```python
from build123d import *

# Parameters (mm, degrees)
SKETCH_1_W      = 60
SKETCH_1_H      = 48
EXTRUDE_1_DEPTH = 36
EXTRUDE_2_REACH = 96.488
SKETCH_2_R      = 10


with BuildPart() as part:
    # 草图1 → 凸台-拉伸1 (new body)
    with BuildSketch(Plane(origin=(0, 0, 0), x_dir=(1, 0, 0), z_dir=(0, 1, 0))):
        Rectangle(SKETCH_1_W, SKETCH_1_H)
    extrude(amount=EXTRUDE_1_DEPTH)

    # 草图2 → 凸台-拉伸2 (add, up to next)
    with BuildSketch(Plane(origin=(54, 0, 0), x_dir=(0, 0, -1), z_dir=(1, 0, 0)), mode=Mode.PRIVATE) as extrude_2_sk1:
        with Locations((0, 18)):
            Circle(SKETCH_2_R)
    extrude_2_tool1 = extrude(extrude_2_sk1.sketch, amount=-EXTRUDE_2_REACH, mode=Mode.PRIVATE) - part.part
    add(extrude_2_tool1.solids().sort_by_distance((54, 18, 0))[0])


solid = part.part
```
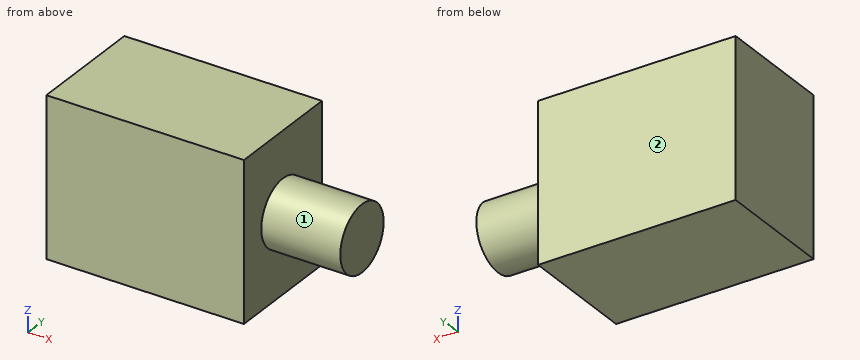
Geometry check sheet. Reference: the model listing, model coordinates, mm. Face numbers are marked on the shaded views. A direction names the side the tool comes from. Round coordinates to 2 decimals unless told otherwise and drop trailing zeros. Order: outer loops, then holes, each group sorted by start corner. A loop starts at its lowest first (then second) coordinate and runs counter-clockwise, first axis right, second up. Notation, with made-up numbers: (-12.5, -28) - (36.5, -28) arc R27 cw to (36.5, -4) - close; hole circle Ø7 at (36.5, 77). An arc over 180 degrees is marked (long way). Use a Markdown table: item, result. Add a question column.
1) Section check A-A (z = 0). Record the cut outline in (x, y), then the cut area to 3 significant figures.
2) Section check C-C (x = 40). Record the cut outline in (y, z), then the cut area to 3 significant figures.
3) Section check D-D (y = 31.5). Record the cut outline in (x, z), then the cut area to 3 significant figures.
4) Gauge pin test, flat ends, axial feed: P1, Ø1, axis at y = 6.5, z = 16, coming from the +X side; P2, Ø11, axis at y = 11.5, z = -9.5, coming from the +X side. Record the tip position at first contact, or that the pin passes through.
5) Set-up check for the marked faces 1 and 2: record each of +Z, -Z, +X, -X, +Y, -Y from which the full face is reachable in a straight line by a thin tool's end or side.
6) Section check B-B (y = 18). Record the cut outline in (x, z).
7) Thickness scan on line 1 along X through (y, z) = (25, -18.5); line 2 along Y through (x, z) = (49.5, -2); line 3 along Y through (x, z) = (33, 4). Record the ranges inside material, lowest first.
Established:
| question | item | result |
|---|---|---|
| 1 | outline | (-30, 0) - (30, 0) - (30, 8) - (54, 8) - (54, 28) - (30, 28) - (30, 36) - (-30, 36) - close |
| 1 | area | 2,640 mm2 |
| 2 | outline | circle Ø20 at (18, 0) |
| 2 | area | 314 mm2 |
| 3 | outline | (-30, -24) - (30, -24) - (30, 24) - (-30, 24) - close |
| 3 | area | 2,880 mm2 |
| 4 | P1 | x = 30 |
| 4 | P2 | x = 54 |
| 5 | face 1 | +X |
| 5 | face 2 | +Z, -Z, +X, -X, +Y |
| 6 | outline | (-30, -24) - (30, -24) - (30, -10) - (54, -10) - (54, 10) - (30, 10) - (30, 24) - (-30, 24) - close |
| 7 | line 1 | -30 to 30 |
| 7 | line 2 | 8.2 to 27.8 |
| 7 | line 3 | 8.83 to 27.17 |
